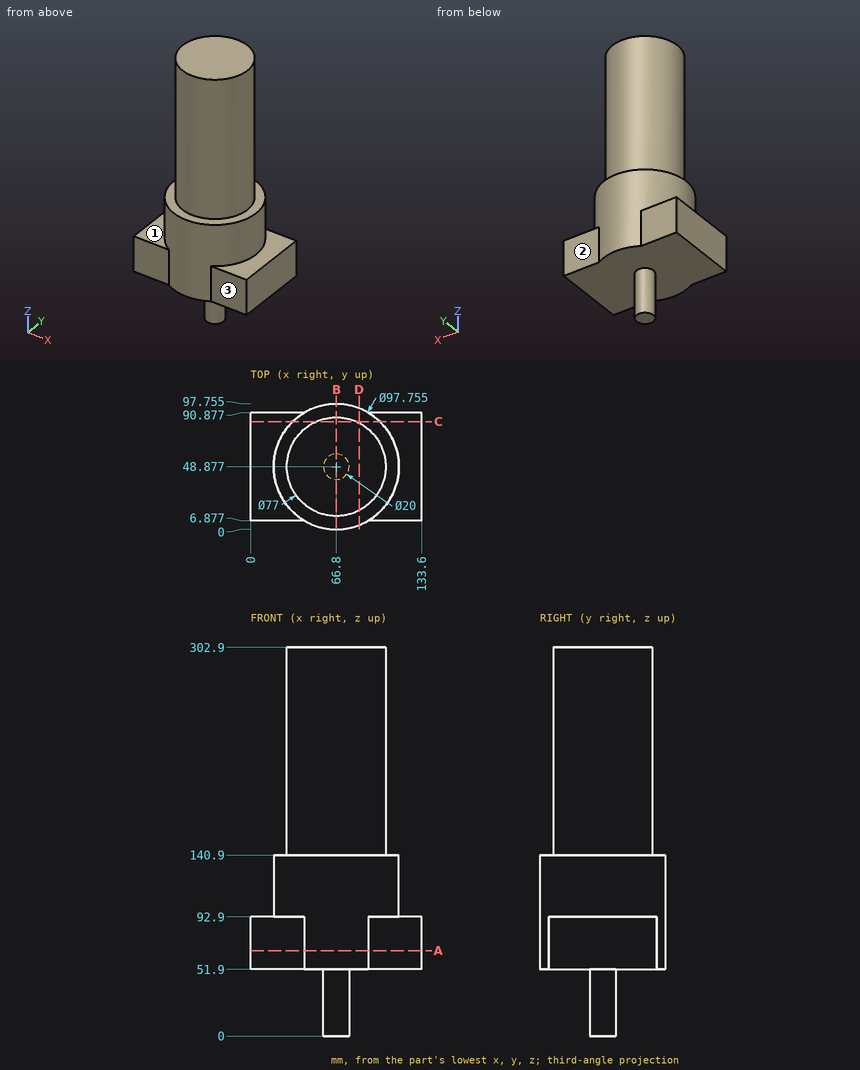
Part print with two shaded views. Sizes in mm from the minimum x, y, z corner. A direction names the side the tool comes from. Coordinates: 2 decimals unless noted, no trailing zeros. Loops run counter-clockwise (first coordinate to the right, second up) from the corner with the lowest first, then second, coordinate; pieces in that order, holes last. Notation, with made-up numbers: (52, 49) - (57, 49) arc R28 ccw to (57, 74) - close; hole circle Ø8 at (73, 21.5). An arc over 180 degrees is marked (long way). Write each question's results on one line, items separated by ' | '. Start each with the question number.
Q1. Slice it at B-B on x = 66.8. Give the cut face in (y, z) (1 decimal), and give its area (3 significant figures).
Q2. Slice it at A-A on z = 66.5. Give the cut face in (x, y) (1 decimal).
Q3. Slice it at C-C on y = 84. Give the cut face in (x, z), and give its area (4 significant figures).
Q4. Which spindle directions (+Z, -Z, +X, -X, +Y, -Y) get a long thin tool onto all of the face, cutting with end or side? Do the marked faces 1, 2 and 3. Say none if no direction does.
Q5. Slice it at D-D on x = 84.5. Give the cut face in (y, z), and give its area (3 significant figures).
Q6. Drop flat-ended pins along their axis: pin 1 Ø1.5 at (x, z) = (91, 73.5) entering from +Y; pin 2 Ø4 at (y, z) = (50, 49) entering from -X; pin 3 Ø5 at (y, z) = (37.5, 187) entering from +X. Give the stop position or say it passes through.
Q7. Probe line 1 along Z through (x, y) = (51.5, 92); line 2 along Z through (x, y) = (52, 68); line 3 along X through (y, z) = (50, 242.5). List the from-to ranges inside material, lowest first.
Answer:
1) outline: (0, 51.9) - (38.9, 51.9) - (38.9, 0) - (58.9, 0) - (58.9, 51.9) - (97.8, 51.9) - (97.8, 140.9) - (87.4, 140.9) - (87.4, 302.9) - (10.4, 302.9) - (10.4, 140.9) - (0, 140.9) - close | area: 22,200 mm2
2) outline: (0, 6.9) - (41.8, 6.9) arc R48.9 ccw to (91.8, 6.9) - (133.6, 6.9) - (133.6, 90.9) - (91.8, 90.9) arc R48.9 ccw to (41.8, 90.9) - (0, 90.9) - close
3) outline: (0, 51.9) - (133.6, 51.9) - (133.6, 92.9) - (100.79, 92.9) - (100.79, 140.9) - (82.57, 140.9) - (82.57, 302.9) - (51.03, 302.9) - (51.03, 140.9) - (32.81, 140.9) - (32.81, 92.9) - (0, 92.9) - close | area: 13,850 mm2
4) face 1: +Z, -X | face 2: +Z, -Z, +X, +Y | face 3: +Z, -Z, +X, -Y
5) outline: (3.32, 51.9) - (94.44, 51.9) - (94.44, 140.9) - (83.07, 140.9) - (83.07, 302.9) - (14.69, 302.9) - (14.69, 140.9) - (3.32, 140.9) - close | area: 19,200 mm2
6) pin 1: stops at y = 91.76 | pin 2: stops at x = 56.8 | pin 3: stops at x = 104.26
7) line 1: z = 51.9 to 140.9 | line 2: z = 51.9 to 302.9 | line 3: x = 28.32 to 105.28
